The listing builds one solid part. Answer for the finished solid, in the listing's coordinates (mm). A direction names the side the tool comes from. Coordinates: 2 decimals unless noted, no trailing zeros.
(1) Given P1, Ø12.5, axis at x = 345.93, y = 10.58, coming from the -Z side; P2, Ø10, axis at x = 530.08, z = -12.7, coming from the -Y side, each flat-ended and moving along its own axis, determine where each tip first touches the part or whether it passes through.
(2) Straight lines are drawn through the part: line 1 (Y direction, x = 382, z = -5.25); line 2 (Z direction, x = 545, y = 15.5) (3 decimals); line 3 (Y direction, x = 122, z = 0.25). For each, find the intervals that lie inside material, in ascending order.
(3) For a pull along Y with two mould halves and no side action, classify faces 3 (the flat face through (872.98, 9, 1)), 4 (the flat face through (438, -4.027, -14)), 5 (the flat face through (438, 24.548, -14)), 6 (the flat face through (438, 21.373, -14)) as +Y half, -Y half, draft (parallel to the pull), parting line (faces both ways), or undercut.
(4) Which of the six approach directions +Z, -Z, +X, -X, +Y, -Y give full straight-line access (tool end or side, diameter ignored) to faces 1 (the flat face through (438, 9, 0)), 2 (the flat face through (14.98, 8, 1))?
from build123d import *

# Parameters (mm, degrees)
SKETCH1_W          = 889
SKETCH1_H          = 31.75
EXTRUDE1_DEPTH     = 28.575
EXTRUDE2_REACH     = 891
SKETCH2_W          = 25.4
SKETCH2_H          = 25.4
HOLE1_D            = 6.35
HOLE1_DEPTH        = 3.175
LPATTERN1_COUNT    = 35
LPATTERN1_PITCH    = 25.4
HOLE2_D            = 9.652
HOLE2_DEPTH        = 3.175
LPATTERN2_COUNT    = 12
LPATTERN2_PITCH    = 25.4
HOLE3_D            = 9.652
HOLE3_DEPTH        = 3.175
HOLE4_D            = 9.652
HOLE4_DEPTH        = 3.175
LPATTERN3_COUNT    = 12
LPATTERN3_PITCH    = 25.4
HOLE5_D            = 3.175
HOLE5_DEPTH        = 3.175
HOLE6_D            = 6.35
HOLE6_DEPTH        = 3.175
LPATTERN4_COUNT    = 35
LPATTERN4_PITCH    = 25.4
FILLET1_R          = 3.175
FILLET2_R          = 3.175
FILLET3_R          = 6.35
FILLET4_R          = 6.35
SKETCH16_R         = 3.175
SKETCH16_W         = 31
SKETCH16_H         = 22.225
CUT_EXTRUDE2_DEPTH = 55


with BuildPart() as part:
    # Sketch1 → Extrude1 (new body)
    with BuildSketch(Plane.XY.offset(3.175)):
        with Locations((428.480011997, 8.672957166)):
            Rectangle(SKETCH1_W, SKETCH1_H)
    extrude(amount=-EXTRUDE1_DEPTH)

    # Sketch2 → Extrude2 (cut, up to next)
    with BuildSketch(Plane.ZY.offset(16.019988003), mode=Mode.PRIVATE) as extrude2_sk1:
        with Locations((-12.7, 8.672957166)):
            Rectangle(SKETCH2_W, SKETCH2_H)
    extrude2_tool1 = extrude(extrude2_sk1.sketch, amount=-EXTRUDE2_REACH, mode=Mode.PRIVATE) & part.part
    add(extrude2_tool1.solids().sort_by_distance((-16.019988, 8.672957, -12.7))[0], mode=Mode.SUBTRACT)

    # Hole1
    with Locations(Plane(origin=(0, 24.547957166, 0), x_dir=(-1, 0, 0), z_dir=(0, 1, 0))):
        with Locations((3.319988003, -12.7)):
            hole1 = Hole(HOLE1_D / 2, depth=HOLE1_DEPTH)

    # LPattern1: Hole1 ×35
    with Locations(*[(i * LPATTERN1_PITCH, 0, 0) for i in range(1, LPATTERN1_COUNT)]):
        add(hole1, mode=Mode.SUBTRACT)

    # Hole2
    with Locations(Plane.XY.offset(3.175)):
        with Locations((66.530011997, 10.577957166)):
            hole2 = Hole(HOLE2_D / 2, depth=HOLE2_DEPTH)

    # LPattern2: Hole2 ×12, 8 skipped
    with Locations(*[(i * LPATTERN2_PITCH, 0, 0) for i in range(1, LPATTERN2_COUNT) if i not in (2, 3, 4, 5, 6, 7, 8, 9)]):
        add(hole2, mode=Mode.SUBTRACT)

    # Hole3
    with Locations(Plane.XY.offset(3.175)):
        with Locations((428.480011997, 6.767957166)):
            Hole(HOLE3_D / 2, depth=HOLE3_DEPTH)

    # Hole4
    with Locations(Plane.XY.offset(3.175)):
        with Locations((511.030011997, 10.577957166)):
            hole4 = Hole(HOLE4_D / 2, depth=HOLE4_DEPTH)

    # LPattern3: Hole4 ×12, 8 skipped
    with Locations(*[(i * LPATTERN3_PITCH, 0, 0) for i in range(1, LPATTERN3_COUNT) if i not in (2, 3, 4, 5, 6, 7, 8, 9)]):
        add(hole4, mode=Mode.SUBTRACT)

    # Hole5
    with Locations(Plane.XY.offset(3.175)):
        with Locations((669.780011997, 8.672957166)):
            Hole(HOLE5_D / 2, depth=HOLE5_DEPTH)

    # Hole6
    with Locations(Plane(origin=(0, -4.027042834, 0), x_dir=(-1, 0, 0), z_dir=(0, 1, 0))):
        with Locations((3.319988003, -12.7)):
            hole6 = Hole(HOLE6_D / 2, depth=HOLE6_DEPTH)

    # LPattern4: Hole6 ×35
    with Locations(*[(i * LPATTERN4_PITCH, 0, 0) for i in range(1, LPATTERN4_COUNT)]):
        add(hole6, mode=Mode.SUBTRACT)

    # Fillet1
    fillet1_edges = [part.edges().sort_by_distance(p)[0] for p in [
        (428.480011997, 21.372957166, 0),
    ]]
    fillet(fillet1_edges, radius=FILLET1_R)

    # Fillet2
    fillet2_edges = [part.edges().sort_by_distance(p)[0] for p in [
        (428.480011997, -4.027042834, 0),
    ]]
    fillet(fillet2_edges, radius=FILLET2_R)

    # Fillet3
    fillet3_edges = [part.edges().sort_by_distance(p)[0] for p in [
        (428.480011997, -7.202042834, 3.175),
    ]]
    fillet(fillet3_edges, radius=FILLET3_R)

    # Fillet4
    fillet4_edges = [part.edges().sort_by_distance(p)[0] for p in [
        (428.480011997, 24.547957166, 3.175),
    ]]
    fillet(fillet4_edges, radius=FILLET4_R)

    # Sketch16 → Cut-Extrude2 (cut)
    with BuildSketch(Plane(origin=(0, 24.547957166, 0), x_dir=(1, 0, 0), z_dir=(0, 1, 0))):
        Polygon((14.980011997, -46.104803879), (14.980011997, 3.175), (-16.019988003, 3.175), (-16.019988003, 25.4), (-32.780059235, 25.4), (-32.780059235, -46.104803879), align=None)
        with Locations((-3.319988003, 12.7)):
            Circle(SKETCH16_R)
        with Locations((-0.519988003, 14.2875)):
            Rectangle(SKETCH16_W, SKETCH16_H)
        with Locations((-3.319988003, 12.7)):
            Circle(SKETCH16_R, mode=Mode.SUBTRACT)
    extrude(amount=-CUT_EXTRUDE2_DEPTH, mode=Mode.SUBTRACT)


solid = part.part
Model answer:
1. P1: stops at z = 0
1. P2: stops at y = -7.2
2. line 1: y = -7.2 to -4.03, 21.37 to 24.55
2. line 2: z = 0 to 3.175
2. line 3: y = -6.2 to 23.55
3. face 3: draft
3. face 4: undercut
3. face 5: +Y half
3. face 6: undercut
4. face 1: -Z, +X, -X
4. face 2: +Z, -Z, -X, +Y, -Y
